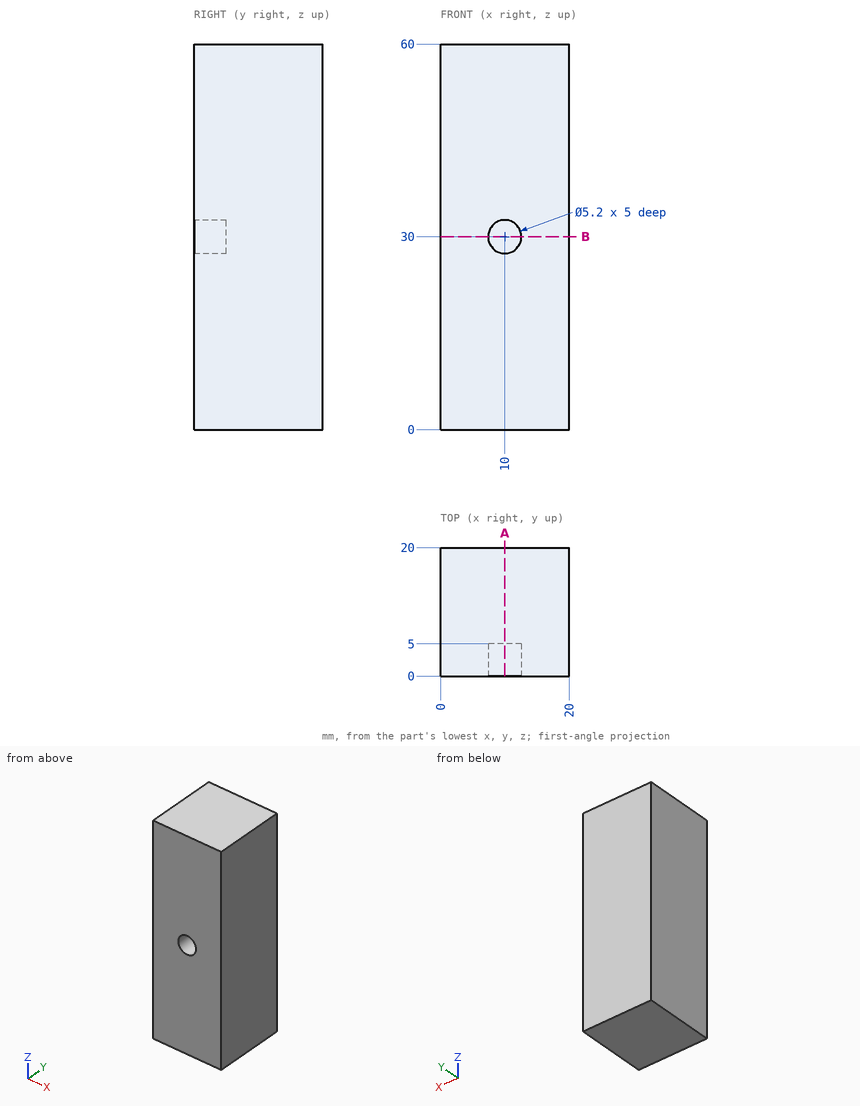
Answer from the drawing. Dimensions are ordinates in mm from the lowest x, y and z of the part. Round coordinates to 2 decimals unless told otherwise and drop trailing zeros. Write each loop counter-clockwise with the first axis right and the second up, starting at its lowest first coordinate (ties: lowest second). Pieces come first, ordered by that corner, then holes.
1. Given pin 1 Ø1.6 at (x, z) = (11, 31) entering from -Y, flat-ended and moving along its own axis, determine where the tip first touches the part or whether it passes through.
2. The part is cut by section B-B, the plane z = 30. Determine the outline of the cut face in (x, y).
3. The part is cut by section A-A, the plane x = 10. Determine the outline of the cut face in (y, z).
4. Straight lines are drawn through the part: L1, parallel to X at y = 3.85, z = 30; L2, parallel to X at y = 3, z = 31. For each, find the intervals that lie inside material, in ascending order.
Values:
1. pin 1: stops at y = 5
2. outline: (0, 0) - (7.4, 0) - (7.4, 5) - (12.6, 5) - (12.6, 0) - (20, 0) - (20, 20) - (0, 20) - close
3. outline: (0, 0) - (20, 0) - (20, 60) - (0, 60) - (0, 32.6) - (5, 32.6) - (5, 27.4) - (0, 27.4) - close
4. L1: x = 0 to 7.4, 12.6 to 20
4. L2: x = 0 to 7.6, 12.4 to 20
